Geometry check sheet. Reference: the model listing, model coordinates, mm. Face numbers are marked on the shaded views. A direction names the side the tool comes from. Give positions to 0.01 mm unless a question says otherwise; leave off trailing zeros. Order: outer loops, then holes, each group sorted by start corner. A loop starts at its lowest first (then second) coordinate and runs counter-clockwise, first axis right, second up. Notation, with made-up numbers: M -30.5,82.5 L 0.5,82.5 A34 ccw 0.5,113.5 Z; hole C 19.5,79 d11. An arc over 180 degrees is marked long. Put each result on its own line as item: value. Start each with the question number.
Q1. Access from +Z, -Z, +X, -X, +Y, -Y to the whole of each face (thin tool, end or side, straight path). Record for the marked faces 5 and 6.
Q2. Section check B-B on x = 10.75. State how many separate pieces and enclosed holes the cut face has, then the cut area to 3 significant figures.
Q3. Go/stop test with flat-tipped pins: pin 1 (1 mm diameter, centred on x = 6, z = 22.5, fed in from -Y); pin 2 (2 mm diameter, centred on x = 1.5, z = 21.5, fed in from -Y). Record where each tip stops, or that it passes through.
Q4. Material ranges on L1, parallel to Z at x = 1.25, y = -13 (3 decimals); L2, parallel to Y at x = 8.75, z = -1; L3, parallel to Z at x = 9.25, y = -4.5 (3 decimals), recorded low to high.
Q5. Section check D-D on z = 29. Record the cut outline in (x, y), then the cut area to 3 significant figures.
Q6. Section check A-A on y = 38.1. Record the cut outline in (x, z) (3 decimals), then the cut area to 3 significant figures.
Q7. Section check C-C on y = -13. Record the cut outline in (x, z) (3 decimals), then the cut area to 3 significant figures.
Q8. Mould release check, pull along Z, two halves, no side actions. Record for the marked faces 1, 2, 3 and 4: +Z half, -Z half, draft (parallel to the pull), parting line (faces both ways), or undercut.
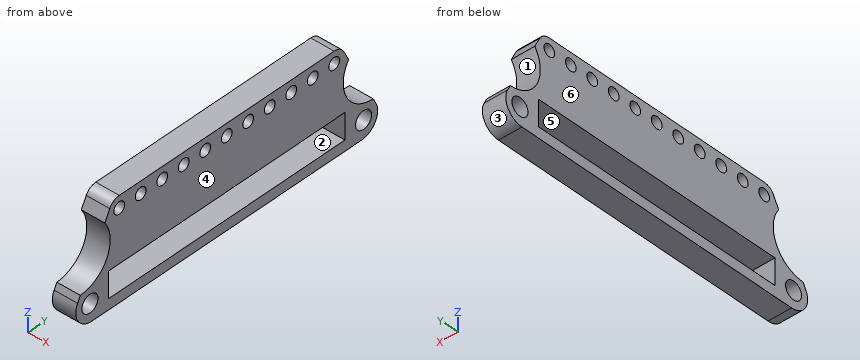
```python
from build123d import *

# Parameters (mm, degrees)
F0_R     = 4.7625
F0_W     = 139.7
F0_H     = 13.97
F0_R_2   = 3.175
F1_DEPTH = 12.7
F3_DEPTH = 25.4
F4_R     = 3.175
F5_DEPTH = 25.4


with BuildPart() as f1:
    # F0 (on Right) → F1 (new body)
    with BuildSketch(Plane.YZ):
        with BuildLine():
            Line((-79.661611154, -12.7), (79.661611154, -12.7))
            ThreePointArc((79.661611154, -12.7), (87.7894077283, -8.1413414953), (88.1372885066, 1.1710923155))
            Line((88.1372885066, 1.1710923155), (69.1504515684, 38.1989076845))
            ThreePointArc((69.1504515684, 38.1989076845), (66.8108943302, 40.720043857), (63.5, 41.6515128075))
            Line((63.5, 41.6515128075), (-63.5, 41.6515128075))
            ThreePointArc((-63.5, 41.6515128075), (-66.8108943302, 40.720043857), (-69.1504515684, 38.1989076845))
            Line((-69.1504515684, 38.1989076845), (-88.1372885066, 1.1710923155))
            ThreePointArc((-88.1372885066, 1.1710923155), (-87.7894077283, -8.1413414953), (-79.661611154, -12.7))
        make_face()
        with Locations((-80.8408441287, -3.175)):
            Circle(F0_R, mode=Mode.SUBTRACT)
        Rectangle(F0_W, F0_H, mode=Mode.SUBTRACT)
        with Locations((80.8408441287, -3.175)):
            Circle(F0_R, mode=Mode.SUBTRACT)
        with Locations((-63.5, 35.3015128075)):
            Circle(F0_R_2, mode=Mode.SUBTRACT)
        with Locations((63.5, 35.3015128075)):
            Circle(F0_R_2, mode=Mode.SUBTRACT)
    extrude(amount=F1_DEPTH)

    # F2 (on face) → F3 (cut)
    with BuildSketch(Plane.YZ.offset(12.7)):
        with BuildLine():
            Line((-72.0478464454, 32.5484561161), (-86.5348208304, 4.2961982741))
            ThreePointArc((-86.5348208304, 4.2961982741), (-70.8156562853, 14.0762348796), (-72.0478464454, 32.5484561161))
        make_face()
        with BuildLine():
            ThreePointArc((72.0478464454, 32.5484561161), (70.8156562853, 14.0762348796), (86.5348208304, 4.2961982741))
            Line((86.5348208304, 4.2961982741), (72.0478464454, 32.5484561161))
        make_face()
    extrude(amount=-F3_DEPTH, mode=Mode.SUBTRACT)

    # F4 (on face) → F5 (cut)
    with BuildSketch(Plane.YZ.offset(12.7)):
        with Locations((-50.8, 35.3015128075)):
            Circle(F4_R)
        with Locations((-38.1, 35.3015128075)):
            Circle(F4_R)
        with Locations((-25.4, 35.3015128075)):
            Circle(F4_R)
        with Locations((-12.7, 35.3015128075)):
            Circle(F4_R)
        with Locations((0, 35.3015128075)):
            Circle(F4_R)
        with Locations((12.7, 35.3015128075)):
            Circle(F4_R)
        with Locations((25.4, 35.3015128075)):
            Circle(F4_R)
        with Locations((38.1, 35.3015128075)):
            Circle(F4_R)
        with Locations((50.8, 35.3015128075)):
            Circle(F4_R)
        with Locations((63.5, 35.3015128075)):
            Circle(F4_R)
    extrude(amount=-F5_DEPTH, mode=Mode.SUBTRACT)


solid = f1.part
```
Results found:
1. face 5: +X, -X
1. face 6: +Z, -Z, -X, +Y, -Y
2. separate pieces: 1
2. enclosed holes: 14
2. area: 5,850 mm^2
3. pin 1: stops at y = -68.85
3. pin 2: stops at y = -68.92
4. L1: z = -12.7 to -6.985, 6.985 to 32.141, 38.462 to 41.652
4. L2: y = -88.93 to -85.08, -76.6 to -69.85, 69.85 to 76.6, 85.08 to 88.93
4. L3: z = -12.7 to -6.985, 6.985 to 41.652
5. outline: M 0,-70.13 L 12.7,-70.13 L 12.7,70.13 L 0,70.13 Z
5. area: 1,780 mm^2
6. outline: M 0,-12.7 L 12.7,-12.7 L 12.7,-6.985 L 0,-6.985 Z; M 0,6.985 L 12.7,6.985 L 12.7,32.127 L 0,32.127 Z; M 0,38.477 L 12.7,38.477 L 12.7,41.652 L 0,41.652 Z
6. area: 432 mm^2
7. outline: M 0,-12.7 L 12.7,-12.7 L 12.7,-6.985 L 0,-6.985 Z; M 0,6.985 L 12.7,6.985 L 12.7,32.141 L 0,32.141 Z; M 0,38.462 L 12.7,38.462 L 12.7,41.652 L 0,41.652 Z
7. area: 433 mm^2
8. face 1: undercut
8. face 2: undercut
8. face 3: parting line
8. face 4: draft
